```python
from build123d import *

# Parameters (mm, degrees)
SKETCH1_R           = 29.060848553
BOSS_EXTRUDE1_DEPTH = 20
SKETCH2_W           = 20
SKETCH2_H           = 12
BOSS_EXTRUDE2_DEPTH = 139.5
FILLET2_R           = 10
BOSS_EXTRUDE3_DEPTH = 12
BOSS_EXTRUDE4_START = 12
BOSS_EXTRUDE4_DEPTH = 12
BOSS_EXTRUDE6_DEPTH = 20


with BuildPart() as part:
    # Sketch1 → Boss-Extrude1 (new body)
    with BuildSketch(Plane.XY):
        Circle(SKETCH1_R)
    extrude(amount=-BOSS_EXTRUDE1_DEPTH)

    # Sketch2 → Boss-Extrude2 (add)
    with BuildSketch(Plane(origin=(0, 0, -20), x_dir=(-1, 0, 0), z_dir=(0, 0, -1))):
        Rectangle(SKETCH2_W, SKETCH2_H)
    extrude(amount=-BOSS_EXTRUDE2_DEPTH)

    # Fillet2
    # the kernel refuses this fillet: 10 mm, written as the material it takes off along each edge
    with BuildSketch(Plane(origin=(10, -31, 119.5), x_dir=(0, 0, -1), z_dir=(0, 1, 0)), Plane(origin=(-10, 31, 119.5), x_dir=(0, 0, -1), z_dir=(0, -1, 0))) as fillet2_piece_1:
        with BuildLine():
            CenterArc((FILLET2_R, FILLET2_R), FILLET2_R, 180, 90)
            Line((0, FILLET2_R), (0, 0))
            Line((0, 0), (FILLET2_R, 0))
        make_face()
    extrude(amount=62, mode=Mode.SUBTRACT)

    # Sketch3 → Boss-Extrude3 (add)
    with BuildSketch(Plane.XZ.offset(6)):
        with BuildLine():
            Line((6.20869835, 102.749264082), (80.315076986, 166.416639129))
            ThreePointArc((80.315076986, 166.416639129), (81.332881571, 179.849603019), (67.899917681, 180.867407604))
            Line((67.899917681, 180.867407604), (-6.206460955, 117.200032557))
            ThreePointArc((-6.206460955, 117.200032557), (-7.224082117, 103.769489485), (6.206460955, 102.751868323))
            Line((6.206460955, 102.751868323), (6.20869835, 102.749264082))
        make_face()
    extrude(amount=BOSS_EXTRUDE3_DEPTH)

    # Sketch4 → Boss-Extrude4 (add)
    with BuildSketch(Plane(origin=(0, -6, 0), x_dir=(1, 0, 0), z_dir=(0, 1, 0)).offset(BOSS_EXTRUDE4_START)):
        with BuildLine():
            Line((72.601205927, -183.04794218), (169.39785175, -198.549240748))
            ThreePointArc((169.39785175, -198.549240748), (180.31006197, -190.649613341), (172.410434564, -179.737403121))
            Line((172.410434564, -179.737403121), (75.613788741, -164.236104553))
            ThreePointArc((75.613788741, -164.236104553), (64.70157852, -172.13573196), (72.601205927, -183.04794218))
        make_face()
    extrude(amount=-BOSS_EXTRUDE4_DEPTH)

    # Sketch5 → Boss-Extrude6 (add)
    with BuildSketch(Plane.XZ.offset(6)):
        with BuildLine():
            Line((161.378376914, 189.143321934), (161.378376914, 73.343321934))
            ThreePointArc((161.378376914, 73.343321934), (170.904143157, 63.817555691), (180.429909401, 73.343321934))
            Line((180.429909401, 73.343321934), (180.429909401, 189.143321934))
            ThreePointArc((180.429909401, 189.143321934), (170.904143157, 198.669088178), (161.378376914, 189.143321934))
        make_face()
    extrude(amount=BOSS_EXTRUDE6_DEPTH)


solid = part.part
```
Could you check a few things on this model? Use its own coordinates, in mm. A direction names the side the tool comes from. Round coordinates to 2 decimals unless told otherwise and drop trailing zeros. Write each loop counter-clockwise with the first axis right and the second up, starting at its lowest first coordinate (ties: lowest second). Pieces come first, ordered by that corner, then holes. Notation, with made-up numbers: M -1,32.25 L 26,32.25 A9 ccw 26,37.25 Z; hole C 70.25,86 d7. An arc over 180 degrees is marked long. Answer in a Markdown table with one row per item. Add a question column.
Q1. On a 3-axis mill with a long thin cutter (end or side, diameter ignored), from which of +Z, -Z, +X, -X, +Y, -Y can I reach the whole of each face in a straight line? I mean faces 1 (the flat face through (37, -18, 139)), 2 (the flat face through (0, 6, 59)), 3 (the flat face through (171, -6, 127)), 4 (the cylindrical face through (-7.36, -11.92, 103.93)), 5 (the cylindrical face through (0.2, 0.1, 119.5)). Say none if no direction works.
Q2. Imagine slicing it at A-A (z = 82). Please give me the cut outline in (x, y), then the cut area to 3 significant figures.
Q3. If we mould it in two halves opening along X, with no side actions, what happens to faces 6 (the flat face through (124.69, 0.084, 172.095)), 7 (the cylindrical face through (13.41, -25.78, -9.86)), 8 (the flat face through (120, -6, 181)), 9 (the flat face through (0, 0, -20))? For each: +X half, -X half, draft (parallel to the pull), parting line (faces both ways), or undercut.
Q4. Imagine slicing it at C-C (x = 0). Please give me the cut outline in (y, z).
Q5. Imagine slicing it at D-D (z = 22). Please give me the cut outline in (x, y), then the cut area to 3 significant figures.
Q6. Will these pins go through, and if not, where does the flat tip stop? pin 1 Ø6 at (x, z) = (-2, 69) entering from +Y; pin 2 Ø17.5 at (x, y) = (3, 4) entering from +Z; pin 3 Ø3 at (x, z) = (16.5, 127.5) entering from +Y.
Q7. Imagine slicing it at B-B (y = 0). Please give me the cut outline in (x, z).
Q8. If I drill on line 1 (Y direction, x = 169, z = 161.5); line 2 (Z direction, x = 10.5, y = -23); line 3 (X direction, y = -12.5, z = 80), over which ranges is the centre line in solid material (lowest first)? Write a range as from..to.
Values:
| question | item | result |
|---|---|---|
| 1 | face 1 | +Z, -X, -Y |
| 1 | face 2 | +Z, +X, -X, +Y |
| 1 | face 3 | -Z, +X, +Y |
| 1 | face 4 | -Y |
| 1 | face 5 | +Z, +Y |
| 2 | outline | M -10,-6 L 10,-6 L 10,6 L -10,6 Z; M 161.38,-26 L 180.43,-26 L 180.43,-6 L 161.38,-6 Z |
| 2 | area | 621 mm^2 |
| 3 | face 6 | +X half |
| 3 | face 7 | parting line |
| 3 | face 8 | undercut |
| 3 | face 9 | draft |
| 4 | outline | M -29.06,-20 L 29.06,-20 L 29.06,0 L 6,0 L 6,119.5 L -6,119.5 L -6,122.53 L -18,122.53 L -18,100.45 L -6,100.45 L -6,0 L -29.06,0 Z |
| 5 | outline | M -10,-6 L 10,-6 L 10,6 L -10,6 Z |
| 5 | area | 240 mm^2 |
| 6 | pin 1 | y = 6 |
| 6 | pin 2 | z = 119.5 |
| 6 | pin 3 | y = -6 |
| 7 | outline | M -29.06,-20 L 29.06,-20 L 29.06,0 L 10,0 L 10,109.5 A10 ccw -10,109.5 L -10,0 L -29.06,0 Z; M 72.6,183.05 A9.53 ccw 75.61,164.24 L 172.41,179.74 A9.53 ccw 169.4,198.55 Z |
| 8 | line 1 | -26..-6 |
| 8 | line 2 | -20..0 |
| 8 | line 3 | 161.38..180.43 |
